Answer from the drawing. Dimensions are ordinates in mm from the lowest x, y and z of the part. Coordinates: 2 decimals unless noted, no trailing zeros. Write each loop counter-clockwise with the first axis right and the second up, starting at its lowest first coordinate (ties: lowest second). Pieces come first, ordered by that corner, then holes. Notation, with made-up numbers: (-32.5, 58) -> (18.5, 58) arc R17 cw to (18.5, 79) -> close; hole circle Ø4 at (66.5, -22). An arc over 180 degrees is marked (long way). Return JSON: item names as keys, results as strings.
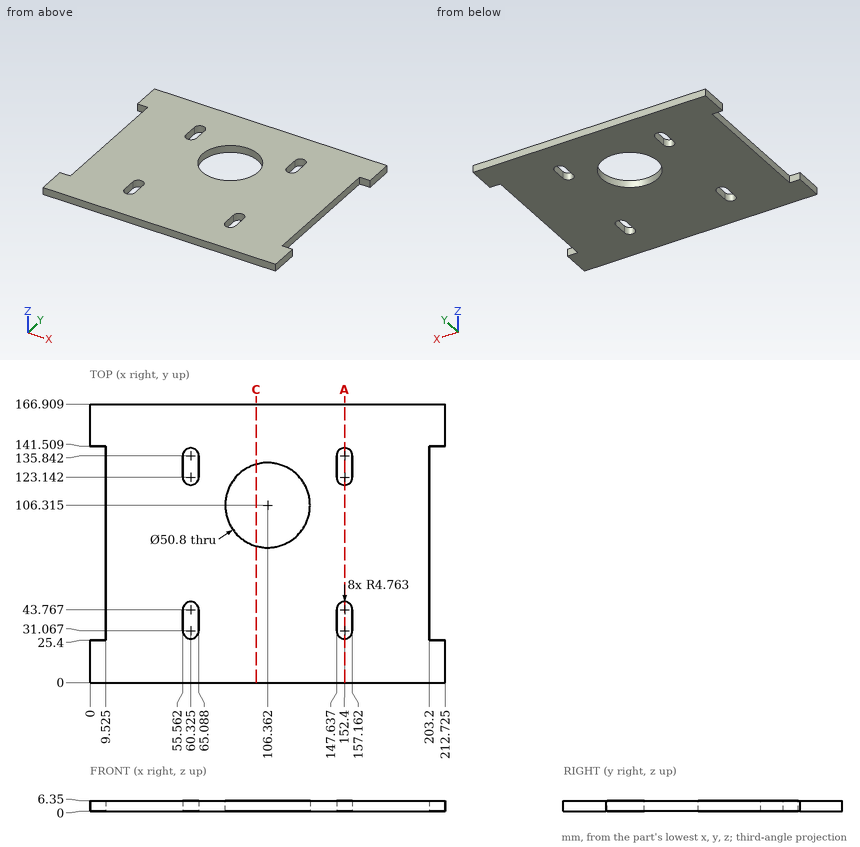
1. Consider L1, parallel to X at y = 33, z = 1.25 (1 decimal); L2, parallel to X at y = 125, z = 1.25 (1 decimal); L3, parallel to X at y = 30, z = 2.5 (1 decimal). Determine where each line is inside the solid, lowest interval first.
Taken from the geometry:
{"L1": "x = 9.5 to 55.6, 65.1 to 147.6, 157.2 to 203.2", "L2": "x = 9.5 to 55.6, 65.1 to 89.2, 123.6 to 147.6, 157.2 to 203.2", "L3": "x = 9.5 to 55.7, 65 to 147.8, 157 to 203.2"}
2. The part is cut by section A-A (x = 152.4). Count the separate pieces of the cut face and the enclosed holes in it.
Taken from the geometry:
{"separate pieces": "3", "enclosed holes": "0"}
3. The part is cut by section C-C (x = 99.5). Determine the outline of the cut face in (y, z).
Taken from the geometry:
{"outline": "(0, 0) -> (81.86, 0) -> (81.86, 6.35) -> (0, 6.35) -> close; (130.77, 0) -> (166.91, 0) -> (166.91, 6.35) -> (130.77, 6.35) -> close"}
4. Flat-ended cylindrical pins translate along their axes: pin 1 Ø1.5 at (x, z) = (73, 2.5) entering from -Y; pin 2 Ø1.5 at (x, y) = (62.5, 139) entering from -Z; pin 3 Ø3 at (y, z) = (130.5, 2) entering from +X; pin 4 Ø3 at (y, z) = (127, 3) entering from -X (1 decimal). Find the tip coordinate at first contact, or state that the pin passes through.
Taken from the geometry:
{"pin 1": "stops at y = 0", "pin 2": "passes through", "pin 3": "stops at x = 203.2", "pin 4": "stops at x = 9.5"}
